from build123d import *

# Parameters (mm, degrees)
CYLINDER1996_R               = 1.5
CYLINDER1996_DEPTH           = 50
COMPOUND1077_PLACEMENT_ANGLE = 225
CYLINDER1997_R               = 1.5
CYLINDER1997_DEPTH           = 50
COMPOUND1078_PLACEMENT_ANGLE = 225
CYLINDER1995_R               = 74
CYLINDER1995_DEPTH           = 40
BOX987_W                     = 42
BOX987_H                     = 10
BOX987_DEPTH                 = 10
COMPOUND1076_PLACEMENT_ANGLE = 225


with BuildPart() as compound1077:
    # Cylinder1996 → Cylinder1996 (new body)
    with BuildSketch(Plane(origin=(9, 100, 59), x_dir=(1, 0, 0), z_dir=(0, -1, 0))):
        Circle(CYLINDER1996_R)
    extrude(amount=CYLINDER1996_DEPTH)


with BuildPart() as compound1077_1:
    # Compound1077 placement: moved
    add(compound1077.part.rotate(Axis((0, 0, 0), (0, 0, 1)), COMPOUND1077_PLACEMENT_ANGLE))


with BuildPart() as compound1079:
    # Cylinder1997 → Cylinder1997 (new body)
    with BuildSketch(Plane(origin=(-9, 100, 59), x_dir=(1, 0, 0), z_dir=(0, -1, 0))):
        Circle(CYLINDER1997_R)
    extrude(amount=CYLINDER1997_DEPTH)


with BuildPart() as compound1079_1:
    # Compound1078 placement: moved
    add(compound1079.part.rotate(Axis((0, 0, 0), (0, 0, 1)), COMPOUND1078_PLACEMENT_ANGLE))

    # Compound1079: union Compound1077
    add(compound1077_1.part)


with BuildPart() as compound1079_2:
    # Compound1079 placement: moved
    add(compound1079_1.part.moved(Location((0, 0, 1))))


with BuildPart() as obj1:
    # Cylinder1995 → Cylinder1995 (new body)
    with BuildSketch(Plane.XY.offset(44)):
        Circle(CYLINDER1995_R)
    extrude(amount=CYLINDER1995_DEPTH)


with BuildPart() as cut673:
    # Box987 → Box987 (new body)
    with BuildSketch(Plane(origin=(-21, -23, 22), x_dir=(1, 0, 0), z_dir=(0, 0, 1))):
        with Locations((21, 5)):
            Rectangle(BOX987_W, BOX987_H)
    extrude(amount=BOX987_DEPTH)


with BuildPart() as cut673_1:
    # Compound1076 placement: moved
    add(cut673.part.moved(Location((63.64, -63.64, 43))).rotate(Axis((63.64, -63.64, 43), (0, 0, 1)), COMPOUND1076_PLACEMENT_ANGLE))

    # Cut672: cut obj1
    add(obj1.part, mode=Mode.SUBTRACT)


with BuildPart() as cut673_2:
    # Cut672 placement: moved
    add(cut673_1.part.moved(Location((0, 0, -10))))

    # Cut673: cut Compound1079
    add(compound1079_2.part, mode=Mode.SUBTRACT)


solid = cut673_2.part
Could you check a few things on this model? Use its own coordinates, in mm. Round coordinates to 2 decimals unless told otherwise and drop trailing zeros. Write each loop counter-clockwise with the first axis right and the second up, starting at its lowest first coordinate (ties: lowest second). Pieces come first, ordered by that corner, then holes. Notation, with made-up numbers: (-20, -2) - (29, -2) arc R19 ccw to (29, 4) - close; hole circle Ø10 at (13.25, 76). An arc over 180 degrees is marked (long way). Put each result on its own line as item: value. Start each with the question number.
(1) Thinking about a two-plate mould opening in Y: for faces 1 (the cylindrical face through (60.563, -45.716, 60.066)), 2 (the cylindrical face through (52.11, -52.54, 59.93)), 3 (the flat face through (37.4, -67.1, 59.9)), which applies, released by +Y, released by -Y, zero draft, split by the parting line, or undercut?
(2) I want a section at B-B, the plane y = -38. Please give me the cut outline in (x, z).
(3) I need wall thicknesses on probe 1 along Z at (x, y) = (59.5, -48.5); probe 2 along X at (y, z) = (-50.5, 58.25); probe 3 along Y at (x, z) = (64, 61). Which ranges of each line are inside material? Lowest first, please.
(4) Will these pins go through, and if not, where does the flat tip stop? pin 1 (6 mm diameter, centred on y = -43, z = 62.5, fed in from -X); pin 2 (1.5 mm diameter, centred on y = -49, z = 62, fed in from +X); pin 3 (3 mm diameter, centred on x = 48.5, z = 63, fed in from +Y).
(5) I want a section at A-A, the plane z = 55.75. Please give me the cut outline in (x, y), plus the area to 3 significant figures.
Here are the results:
1. face 1: undercut
1. face 2: released by +Y
1. face 3: released by -Y
2. outline: (63.5, 55) - (67.7, 55) - (67.7, 65) - (63.5, 65) - close
3. probe 1: z = 55 to 59.13, 60.87 to 65
3. probe 2: x = 54.09 to 58.4
3. probe 3: y = -44.9 to -37.15
4. pin 1: stops at x = 57.97
4. pin 2: stops at x = 60.65
4. pin 3: stops at y = -54.55
5. outline: (35.33, -65.02) - (39.6, -69.3) - (69.3, -39.6) - (65.02, -35.33) arc R74 cw to start
5. area: 168 mm^2
